```python
from build123d import *

# Parameters (mm, degrees)
F0_W     = 111.2547814846
F0_H     = 67.745693028
F1_DEPTH = 50.8
F3_DEPTH = 127
F4_DEPTH = 25.4
F6_DEPTH = 25.4
F7_R     = 10.2195358779
F8_DEPTH = 127


with BuildPart() as f1:
    # F0 (on Top) → F1 (new body)
    with BuildSketch(Plane.XY):
        with Locations((1.1680275202, 1.3140328228)):
            Rectangle(F0_W, F0_H)
    extrude(amount=F1_DEPTH)

    # F2 (on face) → F3 (cut)
    with BuildSketch(Plane.XZ.offset(32.5588136911)):
        with BuildLine():
            Line((10.6582669541, 50.8), (-9.7822453827, 50.8))
            ThreePointArc((-9.7822453827, 50.8), (0.4380107857, 47.116543464), (10.6582669541, 50.8))
        make_face()
    extrude(amount=-F3_DEPTH, mode=Mode.SUBTRACT)

    # F2 (on face) → F4 (join)
    with BuildSketch(Plane.XZ.offset(32.5588136911)):
        with BuildLine():
            ThreePointArc((10.6582669541, 50.8), (0.4380107857, 47.116543464), (-9.7822453827, 50.8))
            Line((-9.7822453827, 50.8), (-21.1705304682, 50.8))
            ThreePointArc((-21.1705304682, 50.8), (-0.2920087427, 38.8142078712), (20.5865129828, 50.8))
            Line((20.5865129828, 50.8), (10.6582669541, 50.8))
        make_face()
    extrude(amount=F4_DEPTH)

    # F5 (on face) → F6 (join)
    with BuildSketch(Plane(origin=(0, 35.1868793368, 0), x_dir=(-1, 0, 0), z_dir=(0, 1, 0))):
        with BuildLine():
            Line((-10.6582669541, 50.8), (-17.0911587775, 50.8))
            ThreePointArc((-17.0911587775, 50.8), (-0.7258458063, 41.8226759797), (15.6394671649, 50.8))
            Line((15.6394671649, 50.8), (9.7822453827, 50.8))
            ThreePointArc((9.7822453827, 50.8), (-0.4380107857, 47.116543464), (-10.6582669541, 50.8))
        make_face()
    extrude(amount=F6_DEPTH)

    # F7 (on face) → F8 (cut)
    with BuildSketch(Plane.XY.offset(50.8)):
        with Locations((-38.438539952, 0)):
            Circle(F7_R)
        with Locations((37.2335724533, 0)):
            Circle(F7_R)
    extrude(amount=-F8_DEPTH, mode=Mode.SUBTRACT)


solid = f1.part
```
Could you check a few things on this model? Use its own coordinates, in mm. A direction names the side the tool comes from. Coordinates: 2 decimals unless noted, no trailing zeros. Order: outer loops, then holes, each group sorted by start corner. A loop starts at its lowest first (then second) coordinate and runs counter-clockwise, first axis right, second up. Notation, with made-up numbers: M -23,-20.75 L -14,-20.75 A22 ccw -14,-11.75 Z; hole C 68.25,84.25 d4. An arc over 180 degrees is marked long. Use one line per item in the form item = value. Start each with the question number.
1. Suppose I cut it at D-D on x = 6. Write out the boundary of the cut face in (y, z).
2. Suppose I cut it at C-C on x = -39. Write out the boundary of the cut face in (y, z).
3. We'd pull the mould along Y, two halves only. Please class faces 4 (the cylindrical face through (-48.65, 0.45, 25.76)), 5 (the flat face through (-1, -57.959, 45)), 6 (the flat face through (-54.459, 1, 25)), 7 (the flat face through (0, 35.187, 25)): +Y half, -Y half, draft (parallel to the pull), parting line (faces both ways), or undercut.
4. For pin 1 (15 mm diameter, centred on x = -11, z = 34.5, fed in from +Y); pin 2 (1.5 mm diameter, centred on x = 7.5, y = -46, fed in from -Z); pin 3 (10 mm diameter, centred on x = -39, z = 12, fed in from -Y), each with a flat end and sliding along its axis, tell me the tip position at first contact or that it passes through.
5. Please list where these lines run through material, in increasing order: line 1 (Y direction, x = -14, z = 48); line 2 (Y direction, x = -1, z = 12.5); line 3 (Y direction, x = 41.5, z = 36).
6. Suppose I cut it at A-A on y = 0. Write out the boundary of the cut face in (x, z).
7. Suppose I cut it at B-B on z = 22. Write out the boundary of the cut face in (x, y), then the cut area to 3 significant figures.
8. On a 3-axis mill with a long thin cutter (end or side, diameter ignored), from which of +Z, -Z, +X, -X, +Y, -Y can I reach the whole of each face in a straight line? I mean faces 1 (the cylindrical face through (-0.645, -45.081, 38.817)), 2 (the flat face through (23, 0, 50.8)), 3 (the cylindrical face through (0.998, 47.709, 41.825)). Say none if no direction works.
Geometry says:
q1.outline = M -57.96,39.65 L -32.56,39.65 L -32.56,0 L 35.19,0 L 35.19,42.55 L 60.59,42.55 L 60.59,48.11 L -57.96,48.11 Z
q2.outline = M -32.56,0 L -10.2,0 L -10.2,50.8 L -32.56,50.8 Z; M 10.2,0 L 35.19,0 L 35.19,50.8 L 10.2,50.8 Z
q3.face_4 = undercut
q3.face_5 = -Y half
q3.face_6 = draft
q3.face_7 = +Y half
q4.pin_1 = 35.19
q4.pin_2 = 39.86
q4.pin_3 = -32.56
q5.line_1 = -57.96 to 35.19
q5.line_2 = -32.56 to 35.19
q5.line_3 = -32.56 to -9.29, 9.29 to 35.19
q6.outline = M -54.46,0 L -48.66,0 L -48.66,50.8 L -54.46,50.8 Z; M -28.22,0 L 27.01,0 L 27.01,50.8 L 10.66,50.8 A16.02 cw -9.78,50.8 L -28.22,50.8 Z; M 47.45,0 L 56.8,0 L 56.8,50.8 L 47.45,50.8 Z
q7.outline = M -54.46,-32.56 L 56.8,-32.56 L 56.8,35.19 L -54.46,35.19 Z; hole C -38.44,0 d20.44; hole C 37.23,0 d20.44
q7.area = 6,880 mm^2
q8.face_1 = -Z, -Y
q8.face_2 = +Z, +X, -X, +Y, -Y
q8.face_3 = -Z, +Y
